Autodesk Inventor part; units mm, degrees
ref_plane "YZ Plane" through (0, 0, 0) normal (1, 0, 0) x (0, 1, 0)
ref_plane "XZ Plane" through (0, 0, 0) normal (0, 1, 0) x (-1, 0, 0)
ref_plane "XY Plane" through (0, 0, 0) normal (0, 0, 1) x (1, 0, 0)
sketch "Sketch1" plane through (0, 0, 0) normal (0, 1, 0) x (-1, 0, 0)
  line L0 (0, 0) -> (0, 25.4)
  line L1 (40.64, 25.4) -> (40.64, 12.7)
  line L2 (40.64, 12.7) -> (2.54, 12.7)
  line L3 (0, 25.4) -> (40.64, 25.4)
  line L4 (0, 0) -> (0, -25.4)
  line L5 (0, -25.4) -> (40.64, -25.4)
  line L6 (40.64, -25.4) -> (40.64, -12.7)
  line L7 (40.64, -12.7) -> (2.54, -12.7)
  line L8 (2.54, -12.7) -> (2.54, 12.7)
  dimension "d2" = 38.1
  dimension "d5" = 25.4
  dimension "d8" = 2.54
  dimension "d9" = 38.1
  dimension "d10" = 12.7
  dimension "d11" = 12.7
  dimension "d12" = 25.4
extrude "Extrusion1" add sketch "Sketch1" along normal blind 50.8
fillet "Fillet1" radius 6.35 1 edges at (-2.54, 25.4, -12.7)
fillet "Fillet2" radius 6.35 1 edges at (-2.54, 25.4, 12.7)
fillet "Fillet3" radius 3.175 1 edges at (-40.64, 25.4, -12.7)
fillet "Fillet4" radius 3.175 1 edges at (-40.64, 25.4, 12.7)
properties part number "Hook0"
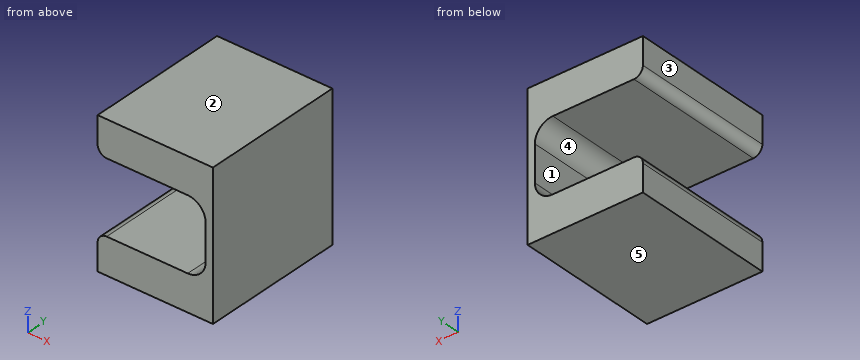
Geometry: final body of the model. Coordinates: model frame, mm. Face numbers are marked on the shaded views. A direction names the side the tool comes from. Round coordinates to 2 decimals unless told otherwise and drop trailing zeros. Order: outer loops, then holes, each group sorted by start corner. A loop starts at its lowest first (then second) coordinate and runs counter-clockwise, first axis right, second up. Notation, with made-up numbers: M -32.75,63.25 L 1.25,63.25 A12 ccw 1.25,73.25 Z; hole C 63,47.5 d6. An arc over 180 degrees is marked long. One line per item, written item: value.
(1) Pull-direction query (Z, two-part tool) for the marked faces 3, 4 and 5; classes: pulls with the +Z half, pulls with the -Z half, needs draft (parallel to the pull), parting line crosses it, or undercut.
Result sheet:
face 3: needs draft
face 4: undercut
face 5: pulls with the -Z half
(2) Pin query (flat end, axial travel): P1, Ø6.5, axis at y = 21, z = 2.5, coming from the -X side. Return the tip coordinate at first contact, or that it passes through.
Result sheet:
P1: x = -2.54
(3) Cut plane B-B (y = 7). Return the cut outline in (x, z) (3 decimals), and give its area (3 significant figures).
Result sheet:
outline: M -40.64,-25.4 L 0,-25.4 L 0,25.4 L -40.64,25.4 L -40.64,15.875 A3.175 ccw -37.465,12.7 L -8.89,12.7 A6.35 cw -2.54,6.35 L -2.54,-6.35 A6.35 cw -8.89,-12.7 L -37.465,-12.7 A3.175 ccw -40.64,-15.875 Z
area: 1,110 mm2
(4) Cut plane C-C (x = -4). Return the cut outline in (y, z), and give its area (3 significant figures).
Result sheet:
outline: M 0,-25.4 L 50.8,-25.4 L 50.8,-10.4 L 0,-10.4 Z; M 0,10.4 L 50.8,10.4 L 50.8,25.4 L 0,25.4 Z
area: 1,520 mm2
(5) Cut plane D-D (z = -14). Return the cut outline in (x, y).
Result sheet:
outline: M -40.03,0 L 0,0 L 0,50.8 L -40.03,50.8 Z
(6) Line query: probe 1 along Z at (x, y) = (-17, 49.5); probe 2 along X at (y, z) = (21, -6); probe 3 along Z at (x, y) = (-7, 32.5). Output: solid intervals per line, ascending. Write a range as [from, to].
Result sheet:
probe 1: [-25.4, -12.7], [12.7, 25.4]
probe 2: [-2.54, 0]
probe 3: [-25.4, -12.41], [12.41, 25.4]
(7) Cut plane A-A (x = -21). Return the cut outline in (y, z).
Result sheet:
outline: M 0,-25.4 L 50.8,-25.4 L 50.8,-12.7 L 0,-12.7 Z; M 0,12.7 L 50.8,12.7 L 50.8,25.4 L 0,25.4 Z
(8) Reachability of the marked faces 1 and 2 from +Z, -Z, +X, -X, +Y, -Y: full face, straight path, thin tool, end or side. Return the list, or none.
Result sheet:
face 1: -X, +Y, -Y
face 2: +Z, +X, -X, +Y, -Y
